Part model, mm, in its own coordinate system. Coordinates: 2 decimals unless noted, no trailing zeros. Loops run counter-clockwise (first coordinate to the right, second up) from the corner with the lowest first, then second, coordinate; pieces in that order, holes last. Notation, with made-up numbers: M 45.25,40.25 L 66.25,40.25 A15 cw 66.25,69.25 Z; hole C 87,-21 d6. An arc over 180 degrees is marked long. Use a Markdown table: item, result. Add a question column.
1) Band-saw the part on B-B (y = 25). List the corners of the cut face in (x, z), plus the area to 4 significant figures.
2) Wall check: probe 1 along X at (y, z) = (45, 3); probe 2 along X at (y, z) = (25, 5.75); probe 3 along Y at (x, z) = (78, 7.75). Give the ranges that are in metal, low to high. Write a range as from..to.
3) Pin check, flat tips, straight feed: pin 1 Ø1.5 at (x, z) = (29.5, 3) entering from -Y; pin 2 Ø3.5 at (x, y) = (-95, 45) entering from -Z; pin 3 Ø2.5 at (x, z) = (87, 5) entering from +Y; pin 4 Ø11.5 at (x, y) = (-82, -39.789) entering from +Z. Stop position of each tip, or through.
4) Band-saw the part on C-C (x = -82). List the corners of the cut face in (y, z), plus the area to 3 significant figures.
5) Band-saw the part on A-A (x = 77). List the corners of the cut face in (y, z), plus the area to 3 significant figures.
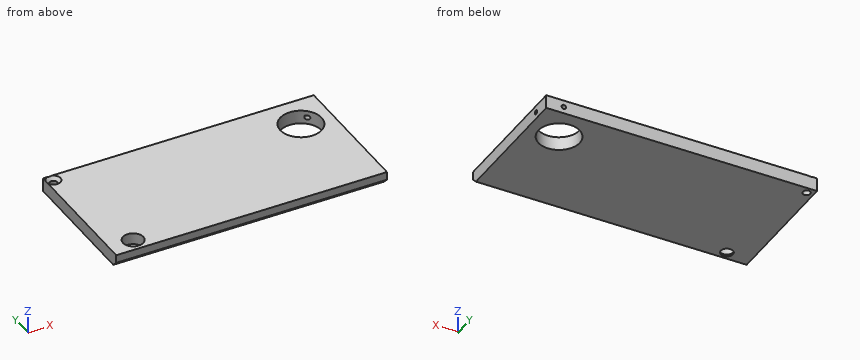
from build123d import *

# Parameters (mm, degrees)
F0_W           = 200
F0_H           = 100
F1_DEPTH       = 10
F2_SIZE        = 4
F4_D           = 9
F4_DEPTH       = 10
F4_CBORE_D     = 15
F4_CBORE_DEPTH = 8.5
F4_TIP         = 2.7038727856
F6_D           = 5.5
F6_DEPTH       = 10
F6_CSINK_D     = 10.4
F6_CSINK_ANGLE = 90
F6_TIP         = 1.6523667023
F8_D           = 30.5
F8_DEPTH       = 10
F8_TIP         = 9.1631244402
F10_D          = 3.3
F10_DEPTH      = 13.6
F10_TIP        = 0.9914200214
F12_D          = 3.3
F12_DEPTH      = 10.1
F12_TIP        = 0.9914200214


with BuildPart() as f1:
    # F0 (on Top) → F1 (new body)
    with BuildSketch(Plane.XY):
        Rectangle(F0_W, F0_H)
    extrude(amount=F1_DEPTH)

    # F2
    f2_edges = [f1.edges().sort_by_distance(p)[0] for p in [
        (0, -50, 0),
    ]]
    chamfer(f2_edges, length=F2_SIZE)

    # F4
    with Locations(Plane.XY.offset(10)):
        with Locations((-82, -39.789)):
            CounterBoreHole(F4_D / 2, F4_CBORE_D / 2, F4_CBORE_DEPTH, depth=F4_DEPTH)
            with Locations((0, 0, -(F4_DEPTH + F4_TIP / 2))):  # 118° drill point
                Cone(0, F4_D / 2, F4_TIP, mode=Mode.SUBTRACT)

    # F6
    with Locations(Plane.XY.offset(10)):
        with Locations((-95, 45)):
            CounterSinkHole(F6_D / 2, F6_CSINK_D / 2, depth=F6_DEPTH, counter_sink_angle=F6_CSINK_ANGLE)
            with Locations((0, 0, -(F6_DEPTH + F6_TIP / 2))):  # 118° drill point
                Cone(0, F6_D / 2, F6_TIP, mode=Mode.SUBTRACT)

    # F8
    with Locations(Plane.XY.offset(10)):
        with Locations((77, 25)):
            Hole(F8_D / 2, depth=F8_DEPTH)
            with Locations((0, 0, -(F8_DEPTH + F8_TIP / 2))):  # 118° drill point
                Cone(0, F8_D / 2, F8_TIP, mode=Mode.SUBTRACT)

    # F10
    with Locations(Plane.YZ.offset(100)):
        with Locations((36, 5)):
            Hole(F10_D / 2, depth=F10_DEPTH)
            with Locations((0, 0, -(F10_DEPTH + F10_TIP / 2))):  # 118° drill point
                Cone(0, F10_D / 2, F10_TIP, mode=Mode.SUBTRACT)

    # F12
    with Locations(Plane(origin=(0, 50, 0), x_dir=(-1, 0, 0), z_dir=(0, 1, 0))):
        with Locations((-87, 5)):
            Hole(F12_D / 2, depth=F12_DEPTH)
            with Locations((0, 0, -(F12_DEPTH + F12_TIP / 2))):  # 118° drill point
                Cone(0, F12_D / 2, F12_TIP, mode=Mode.SUBTRACT)


solid = f1.part
Entries:
| question | item | result |
|---|---|---|
| 1 | outline | M -100,0 L 61.75,0 L 61.75,10 L -100,10 Z; M 92.25,0 L 100,0 L 100,10 L 92.25,10 Z |
| 1 | area | 1,695 mm2 |
| 2 | probe 1 | -100..-97.75, -92.25..100 |
| 2 | probe 2 | -100..61.75, 92.25..100 |
| 2 | probe 3 | -50..9.78, 40.22..50 |
| 3 | pin 1 | y = -49.75 |
| 3 | pin 2 | through |
| 3 | pin 3 | y = 39.66 |
| 3 | pin 4 | z = 1.5 |
| 4 | outline | M -50,4 L -46,0 L -44.29,0 L -44.29,1.5 L -47.29,1.5 L -47.29,10 L -50,10 Z; M -35.29,0 L 50,0 L 50,10 L -32.29,10 L -32.29,1.5 L -35.29,1.5 Z |
| 4 | area | 851 mm2 |
| 5 | outline | M -50,4 L -46,0 L 9.75,0 L 9.75,10 L -50,10 Z; M 40.25,0 L 50,0 L 50,10 L 40.25,10 Z |
| 5 | area | 687 mm2 |
